For this review, take the finished solid that the model builds, in its own axes (mm). Face numbers are marked on the shaded views. A direction names the side the tool comes from. Coordinates: 2 decimals unless noted, no trailing zeros. Loops run counter-clockwise (first coordinate to the right, second up) from the corner with the lowest first, then second, coordinate; pieces in that order, holes last. Notation, with made-up numbers: (30.25, -34.75) -> (75.25, -34.75) arc R6 ccw to (75.25, -26.75) -> close; hole circle Ø11 at (85.25, 88.5). An arc over 180 degrees is marked (long way). Use a Markdown table: item, result.
from build123d import *

# Parameters (mm, degrees)
CROQUIS1_W              = 20
CROQUIS1_H              = 14
SALIENTE_EXTRUIR1_DEPTH = 15
CROQUIS2_W              = 15.6
CROQUIS2_H              = 12.6
CORTAR_EXTRUIR1_DEPTH   = 23.825424421
CROQUIS3_W              = 15
CROQUIS3_H              = 2.5
SALIENTE_EXTRUIR2_DEPTH = 5
CROQUIS4_W              = 15
CROQUIS4_H              = 2.5
SALIENTE_EXTRUIR3_DEPTH = 5
SALIENTE_EXTRUIR4_DEPTH = 0.5


with BuildPart() as part:
    # Croquis1 → Saliente-Extruir1 (new body)
    with BuildSketch(Plane.XY):
        with Locations((0, 7)):
            Rectangle(CROQUIS1_W, CROQUIS1_H)
    extrude(amount=SALIENTE_EXTRUIR1_DEPTH)

    # Croquis2 → Cortar-Extruir1 (cut, through all)
    with BuildSketch(Plane.XY.offset(15)):
        with Locations((0, 6.3)):
            Rectangle(CROQUIS2_W, CROQUIS2_H)
    extrude(amount=-CORTAR_EXTRUIR1_DEPTH, mode=Mode.SUBTRACT)

    # Croquis3 → Saliente-Extruir2 (add)
    with BuildSketch(Plane(origin=(10, 0, 0), x_dir=(0, 0, -1), z_dir=(1, 0, 0))):
        with Locations((-7.5, 1.25)):
            Rectangle(CROQUIS3_W, CROQUIS3_H)
    extrude(amount=SALIENTE_EXTRUIR2_DEPTH)

    # Croquis4 → Saliente-Extruir3 (add)
    with BuildSketch(Plane.ZY.offset(10)):
        with Locations((7.5, 1.25)):
            Rectangle(CROQUIS4_W, CROQUIS4_H)
    extrude(amount=SALIENTE_EXTRUIR3_DEPTH)

    # Croquis5 → Saliente-Extruir4 (add)
    # profile 1 of 3: a face of its own
    with BuildSketch(Plane(origin=(0, 14, 0), x_dir=(1, 0, 0), z_dir=(0, 1, 0))):
        with BuildLine():
            Line((-2.88502332, -10.364727743), (-3.788817138, -10.364727743))
            Line((-3.788817138, -10.364727743), (-5.777163537, -8.035991464))
            Line((-5.777163537, -8.035991464), (-7.016652202, -8.035991464))
            Line((-7.016652202, -8.035991464), (-7.016652202, -10.364727743))
            Line((-7.016652202, -10.364727743), (-7.767857453, -10.364727743))
            Line((-7.767857453, -10.364727743), (-7.767857453, -4.430206259))
            Line((-7.767857453, -4.430206259), (-6.130464757, -4.430206259))
            add(Edge.make_bspline(
                [(-6.130464757, -4.430206259), (-6.0459413, -4.431165013), (-5.883831835, -4.433003829), (-5.651888426, -4.445217717), (-5.441974521, -4.467695996), (-5.251420073, -4.497198358), (-5.076320928, -4.540077128), (-4.911710387, -4.595085737), (-4.756352702, -4.665254498), (-4.659629191, -4.7231034), (-4.61162164, -4.751816007)],
                knots=[0, 0, 0, 0, 1.288415781, 2.47108201, 3.538680541, 4.505415573, 5.408010686, 6.28309489, 7.147834801, 8, 8, 8, 8], degree=3))
            add(Edge.make_bspline(
                [(-4.61162164, -4.751816007), (-4.56060529, -4.787000395), (-4.460070052, -4.856336418), (-4.326599875, -4.980440946), (-4.209578564, -5.1165849), (-4.110973827, -5.26783655), (-4.02967085, -5.435680707), (-3.976798666, -5.62564965), (-3.941292298, -5.835036609), (-3.938280358, -5.98174904), (-3.936710672, -6.058208889)],
                knots=[0, 0, 0, 0, 0.963681284, 1.899076006, 2.827943621, 3.752026167, 4.702860247, 5.71857009, 6.811022445, 8, 8, 8, 8], degree=3))
            add(Edge.make_bspline(
                [(-3.936710672, -6.058208889), (-3.93745934, -6.111069878), (-3.93892671, -6.214676048), (-3.954968911, -6.366794009), (-3.979251178, -6.512331235), (-4.01310717, -6.651852236), (-4.05794689, -6.784371061), (-4.111642187, -6.910836248), (-4.176966463, -7.029766654), (-4.250819351, -7.142352152), (-4.333124618, -7.248469966), (-4.424228497, -7.346918297), (-4.521492422, -7.440360452), (-4.627505642, -7.525742064), (-4.740372634, -7.604737188), (-4.860837683, -7.676024782), (-4.98763716, -7.742797298), (-5.076899105, -7.780006005), (-5.122206459, -7.798892307)],
                knots=[0, 0, 0, 0, 1.126128489, 2.207182719, 3.255820935, 4.268986334, 5.263032379, 6.234153775, 7.193063852, 8.150486488, 9.10116855, 10.051301984, 11.006725633, 11.972966631, 12.949086479, 13.94005042, 14.954415947, 16, 16, 16, 16], degree=3))
            Line((-5.122206459, -7.798892307), (-2.88502332, -10.364727743))
        make_face()
        with BuildLine():
            add(Edge.make_bspline(
                [(-4.763036448, -6.105159217), (-4.76425827, -6.063643734), (-4.766654107, -5.982237185), (-4.782538048, -5.863974915), (-4.811639256, -5.753311079), (-4.849434013, -5.64927727), (-4.902032931, -5.552802913), (-4.968287593, -5.463820517), (-5.050018411, -5.383249363), (-5.113312501, -5.338238747), (-5.145681623, -5.315219945)],
                knots=[0, 0, 0, 0, 1.085368415, 2.128268547, 3.1106313, 4.071895604, 5.014699805, 5.972038339, 6.962883605, 8, 8, 8, 8], degree=3))
            add(Edge.make_bspline(
                [(-5.145681623, -5.315219945), (-5.175015585, -5.296501747), (-5.234192037, -5.258740856), (-5.332300766, -5.214393463), (-5.437527778, -5.177833986), (-5.551527993, -5.151906272), (-5.67362264, -5.129845566), (-5.805927755, -5.117301749), (-5.948364796, -5.106770759), (-6.046712907, -5.10645458), (-6.097599527, -5.106290985)],
                knots=[0, 0, 0, 0, 0.843459406, 1.701540853, 2.6053125, 3.542575708, 4.535326681, 5.614234208, 6.765573065, 8, 8, 8, 8], degree=3))
            Line((-6.097599527, -5.106290985), (-7.016652202, -5.106290985))
            Line((-7.016652202, -5.106290985), (-7.016652202, -7.359906738))
            Line((-7.016652202, -7.359906738), (-6.22671293, -7.359906738))
            add(Edge.make_bspline(
                [(-6.22671293, -7.359906738), (-6.166842369, -7.358806598), (-6.050896861, -7.356676062), (-5.882983115, -7.346006667), (-5.727291264, -7.323687715), (-5.581932855, -7.297806333), (-5.447903419, -7.255709311), (-5.323535107, -7.202662948), (-5.210703341, -7.132400077), (-5.143863862, -7.075910781), (-5.110468877, -7.047687056)],
                knots=[0, 0, 0, 0, 1.210655428, 2.344558938, 3.398352313, 4.389640028, 5.325372474, 6.232137918, 7.116723723, 8, 8, 8, 8], degree=3))
            add(Edge.make_bspline(
                [(-5.110468877, -7.047687056), (-5.081919706, -7.019018524), (-5.025727055, -6.962590938), (-4.955449604, -6.866968879), (-4.894853881, -6.767164245), (-4.845837842, -6.659290565), (-4.807837038, -6.540844414), (-4.781139775, -6.408636819), (-4.766726062, -6.261588504), (-4.764301436, -6.158791145), (-4.763036448, -6.105159217)],
                knots=[0, 0, 0, 0, 0.936271895, 1.842841591, 2.741489519, 3.638077323, 4.58130199, 5.617848582, 6.75717263, 8, 8, 8, 8], degree=3))
        make_face(mode=Mode.SUBTRACT)
    # profile 2 of 3: a face of its own
    with BuildSketch(Plane(origin=(0, 14, 0), x_dir=(1, 0, 0), z_dir=(0, 1, 0))):
        Polygon((1.697328712, -10.364727743), (-2.133818069, -10.364727743), (-2.133818069, -4.430206259), (1.697328712, -4.430206259), (1.697328712, -5.106290985), (-1.382612818, -5.106290985), (-1.382612818, -6.758942537), (1.697328712, -6.758942537), (1.697328712, -7.435027264), (-1.382612818, -7.435027264), (-1.382612818, -9.688643017), (1.697328712, -9.688643017), align=None)
    # profile 3 of 3: a face of its own
    with BuildSketch(Plane(origin=(0, 14, 0), x_dir=(1, 0, 0), z_dir=(0, 1, 0))):
        Polygon((8.157693872, -10.364727743), (7.406488621, -10.364727743), (7.406488621, -5.247141969), (5.790223573, -8.712076191), (5.330110356, -8.712076191), (3.72558289, -5.247141969), (3.72558289, -10.364727743), (2.974377639, -10.364727743), (2.974377639, -4.430206259), (4.057756462, -4.430206259), (5.607117293, -7.720250507), (7.10600652, -4.430206259), (8.157693872, -4.430206259), align=None)
    extrude(amount=SALIENTE_EXTRUIR4_DEPTH)


solid = part.part
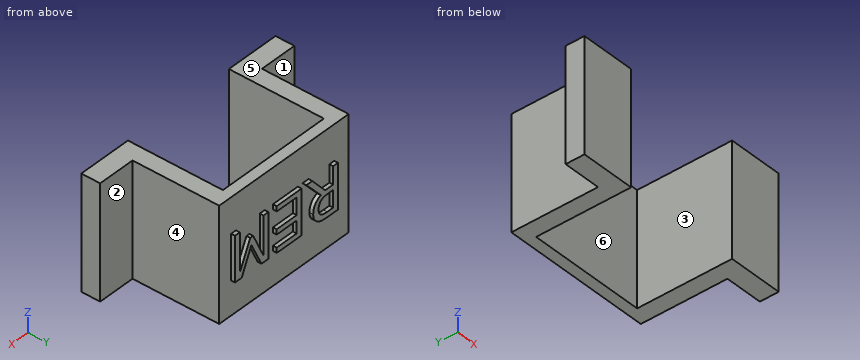
(1) Mouldability with a two-part tool opening along X and no side actions: class the marked faces 4, 5 and 6 as pulls with the +X half, pulls with the -X half, needs draft (parallel to the pull), parting line crosses it, or undercut.
Found:
| item | result |
|---|---|
| face 4 | pulls with the +X half |
| face 5 | needs draft |
| face 6 | undercut |
(2) For line 1 along X through (y, z) = (1, 1); line 2 along X through (y, z) = (3.5, 1); line 3 along Y through (x, z) = (-11.5, 11.75), list the stretches that pass through material, from the lowest coordinate up.
Found:
| item | result |
|---|---|
| line 1 | x = -15 to -7.8, 7.8 to 15 |
| line 2 | x = -10 to -7.8, 7.8 to 10 |
| line 3 | y = 0 to 2.5 |
(3) Take a section at A-A on y = 1.75. Write out the cut boundary in (x, z), plus the area to 3 significant figures.
Found:
| item | result |
|---|---|
| outline | (-15, 0) -> (-7.8, 0) -> (-7.8, 15) -> (-15, 15) -> close; (7.8, 0) -> (15, 0) -> (15, 15) -> (7.8, 15) -> close |
| area | 216 mm^2 |
(4) Take a section at C-C on z = 11. Write out the cut boundary in (x, y).
Found:
| item | result |
|---|---|
| outline | (-15, 0) -> (-7.8, 0) -> (-7.8, 12.6) -> (7.8, 12.6) -> (7.8, 0) -> (15, 0) -> (15, 2.5) -> (10, 2.5) -> (10, 14) -> (-10, 14) -> (-10, 2.5) -> (-15, 2.5) -> close |
(5) Take a section at D-D on y = 6. Write out the cut boundary in (x, z).
Found:
| item | result |
|---|---|
| outline | (-10, 0) -> (-7.8, 0) -> (-7.8, 15) -> (-10, 15) -> close; (7.8, 0) -> (10, 0) -> (10, 15) -> (7.8, 15) -> close |
(6) Take a section at B-B on x = -0.5. Write out the cut boundary in (y, z).
Found:
| item | result |
|---|---|
| outline | (12.6, 0) -> (14, 0) -> (14, 4.43) -> (14.5, 4.43) -> (14.5, 5.11) -> (14, 5.11) -> (14, 6.76) -> (14.5, 6.76) -> (14.5, 7.44) -> (14, 7.44) -> (14, 9.69) -> (14.5, 9.69) -> (14.5, 10.36) -> (14, 10.36) -> (14, 15) -> (12.6, 15) -> close |
(7) For the marked faces 1, 2 and 3, list the 3-axis set-ups (+Z, -Z, +X, -X, +Y, -Y) from which the entire face can be reached by the end or side of a thin tool; tool diameter is ignored.
Found:
| item | result |
|---|---|
| face 1 | +Z, -Z, -X, +Y |
| face 2 | +Z, -Z, +X, +Y |
| face 3 | +Z, -Z, -Y |
(8) For pin 1 Ø1.5 at (y, z) = (5, 6.5) entering from +X; pin 2 Ø5.5 at (x, z) = (-12, 6.5) entering from +Y; pin 3 Ø4.5 at (x, z) = (-1, 4) entering from -Y, all flat-tipped, find the tip position at first contact; note any pin that passes through.
Found:
| item | result |
|---|---|
| pin 1 | stops at x = 10 |
| pin 2 | stops at y = 14 |
| pin 3 | stops at y = 12.6 |
